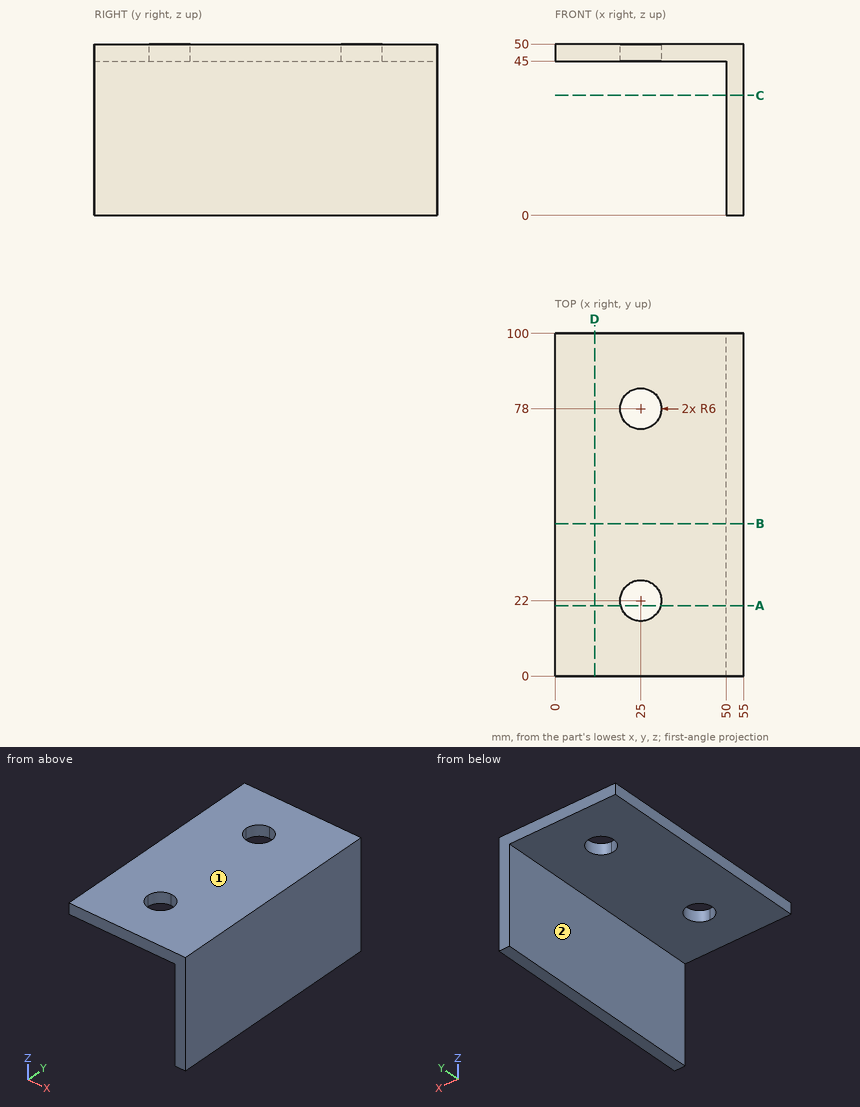
Input: dimensioned drawing with shaded views. Units: mm. Origin: part minimum x, y, z. A direction names the side the tool comes from. Round coordinates to 2 decimals unless told otherwise and drop trailing zeros. Loops run counter-clockwise (first coordinate to the right, second up) from the corner with the lowest first, then second, coordinate; pieces in that order, holes last. Notation, with made-up numbers: M -37.75,24 L -19.75,24 A26 cw -19.75,62 Z; hole C 20.5,65 d1. An arc over 180 degrees is marked long. Return JSON: item names as keys, results as strings. Group by question number.
1. Material intervals for line 1 along X through (y, z) = (20.5, 30.5); line 2 along Z through (x, y) = (31.5, 14.5), sorted ascending. Write a range as from..to.
2. Pin query (flat end, axial travel): pin 1 (2 mm diameter, centred on x = 8, y = 20.5, fed in from -Z); pin 2 (22.5 mm diameter, centred on y = 35, z = 33.5, fed in from -X). Return the tip coordinate at first contact, or that it passes through.
3. Reachability of the marked faces 1 and 2 from +Z, -Z, +X, -X, +Y, -Y: full face, straight path, thin tool, end or side. Return the list, or none.
4. Section query D-D on x = 11.5. Output: boundary loops of the cut face in (y, z).
5. Section query C-C on z = 35. Output: boundary loops of the cut face in (x, y), and give its area (3 significant figures).
6. Section query A-A on y = 20.5. Output: boundary loops of the cut face in (x, z).
7. Section query B-B on y = 44.5. Output: boundary loops of the cut face in (x, z), and give its area (3 significant figures).
Checks:
{
 "1": {"line 1": "x = 50..55", "line 2": "z = 45..50"},
 "2": {"pin 1": "stops at z = 45", "pin 2": "stops at x = 50"},
 "3": {"face 1": "+Z, +X, -X, +Y, -Y", "face 2": "-Z, -X, +Y, -Y"},
 "4": {"outline": "M 0,45 L 100,45 L 100,50 L 0,50 Z"},
 "5": {"outline": "M 50,0 L 55,0 L 55,100 L 50,100 Z", "area": "500 mm²"},
 "6": {"outline": "M 0,45 L 19.19,45 L 19.19,50 L 0,50 Z; M 30.81,45 L 50,45 L 50,0 L 55,0 L 55,50 L 30.81,50 Z"},
 "7": {"outline": "M 0,45 L 50,45 L 50,0 L 55,0 L 55,50 L 0,50 Z", "area": "500 mm²"}
}
